from build123d import *

# Parameters (mm, degrees)
CUT_EXTRUDE1_DEPTH = 2.5


with BuildPart() as part:
    # Sketch1 → Revolve1 (revolve)
    with BuildSketch(Plane(origin=(0, 0, 0), x_dir=(1, 0, 0), z_dir=(0, 1, 0)), mode=Mode.PRIVATE) as revolve1_sk:
        with BuildLine():
            Line((-1.5, 0), (-4, 0))
            Line((-4, 0), (-5.5, 0))
            ThreePointArc((-5.5, 0), (-4.439339828, 0.439339828), (-4, 1.5))
            Line((-4, 1.5), (-4, 7.2))
            Line((-4, 7.2), (-1.5, 7.2))
            Line((-1.5, 7.2), (-1.5, 0))
        make_face()
    revolve(revolve1_sk.sketch.rotate(Axis((0, 0, 0), (0, 0, -1)), 180), axis=Axis((0, 0, 0), (0, 0, -1)))

    # Sketch2 → Cut-Extrude1 (cut)
    with BuildSketch(Plane.XY):
        Polygon((1.674315781, 2.9), (-1.674315781, 2.9), (-3.348631561, 0), (-1.674315781, -2.9), (1.674315781, -2.9), (3.348631561, 0), align=None)
    extrude(amount=-CUT_EXTRUDE1_DEPTH, mode=Mode.SUBTRACT)


solid = part.part
Work out the finished part from the listing and answer in its coordinate system (mm). A direction names the side the tool comes from. Give positions to 0.01 mm unless a question says otherwise; leave off trailing zeros. Write each loop counter-clockwise with the first axis right and the second up, starting at its lowest first coordinate (ties: lowest second). Pieces come first, ordered by that corner, then holes. Notation, with made-up numbers: (4, 60.5) - (48, 60.5) arc R17 cw to (48, 67.5) - close; hole circle Ø8 at (-10, 16.5). An arc over 180 degrees is marked (long way). One line per item, written item: value. Start each with the question number.
1. Find section B-B (z = -1.25). Write down the section's boundary in (x, y), then the cut area to 3 significant figures.
2. Consider probe 1 along Y at (x, z) = (0, -5.7); probe 2 along Z at (x, y) = (-0.5, 2.5); probe 3 along X at (y, z) = (-1.5, -1). Determine where each line is inside the solid, lowest interval first.
3. Find section C-C (z = -3). Write down the section's boundary in (x, y), then the cut area to 3 significant figures.
4. Given pin 1 (0.8 mm diameter, centred on x = -0.5, z = -1, fed in from +Y); pin 2 (3 mm diameter, centred on y = -4, z = -3, fed in from -X); pin 3 (1.5 mm diameter, centred on x = -3.5, y = -4, fed in from -Z), each flat-ended and moving along its own axis, determine where each tip first touches the part or whether it passes through.
5. Find section D-D (z = -0.5). Write down the section's boundary in (x, y), then the cut area to 3 significant figures.
6. For faces 4 (the flat face through (2, 0, -7.2)), 5 (the flat face through (-2.523, -1.43, -1.232)), determine the directions among +Z, -Z, +X, -X, +Y, -Y from which every point of the face is accessible in a straight line to the end or side of a thin tool.
7. Find section A-A (x = 0). Write down the section's boundary in (y, z), then the cut area to 3 significant figures.
8. For a pull along Y with two mould halves and no side action, classify faces 1 (the flat face through (-2.4, 2.4, 0)), 2 (the cylindrical face through (-0.867, 3.905, -4.39)), 3 (the flat face through (-2.5, 1.47, -1.23)) as +Y half, -Y half, draft (parallel to the pull), parting line (faces both ways), or undercut.
Geometry results:
1. outline: circle Ø8.04 at (0, 0); hole (-3.35, 0) - (-1.67, -2.9) - (1.67, -2.9) - (3.35, 0) - (1.67, 2.9) - (-1.67, 2.9) - close
1. area: 21.7 mm2
2. probe 1: -4 to -1.5, 1.5 to 4
2. probe 2: -7.2 to -2.5
2. probe 3: -3.8 to -2.48, 2.48 to 3.8
3. outline: circle Ø8 at (0, 0); hole circle Ø3 at (0, 0)
3. area: 43.2 mm2
4. pin 1: y = 4.27
4. pin 2: x = -3.12
4. pin 3: z = -0.33
5. outline: circle Ø8.76 at (0, 0); hole (-3.35, 0) - (-1.67, -2.9) - (1.67, -2.9) - (3.35, 0) - (1.67, 2.9) - (-1.67, 2.9) - close
5. area: 31.2 mm2
6. face 4: -Z, +X, -X, +Y, -Y
6. face 5: +Z
7. outline: (-5.5, 0) arc R1.5 cw to (-4, -1.5) - (-4, -7.2) - (-1.5, -7.2) - (-1.5, -2.5) - (-2.9, -2.5) - (-2.9, 0) - close; (1.5, -7.2) - (4, -7.2) - (4, -1.5) arc R1.5 cw to (5.5, 0) - (2.9, 0) - (2.9, -2.5) - (1.5, -2.5) - close
7. area: 30.0 mm2
8. face 1: draft
8. face 2: parting line
8. face 3: undercut
